The listing builds one solid part. Answer for the finished solid, in the listing's coordinates (mm). A direction names the side the tool comes from. Coordinates: 2 decimals unless noted, no trailing zeros. Order: outer loops, then holes, each group sorted by start corner. A loop starts at its lowest first (then second) coordinate and runs counter-clockwise, first axis right, second up. Notation, with made-up numbers: (-38.75, -37) -> (2.25, -37) arc R35 ccw to (2.25, -5) -> close; hole circle Ø3 at (38.5, 27.25). An arc over 180 degrees is marked (long way). One line per question, with ' | ' between items.
Autodesk Inventor part; units mm, degrees
ref_plane "YZ Plane" through (0, 0, 0) normal (1, 0, 0) x (0, 1, 0)
ref_plane "XZ Plane" through (0, 0, 0) normal (0, 1, 0) x (-1, 0, 0)
ref_plane "XY Plane" through (0, 0, 0) normal (0, 0, 1) x (1, 0, 0)
sketch "Sketch1" plane through (0, 0, 0) normal (0, 1, 0) x (-1, 0, 0)
  line L0 (0, 0) -> (125, 0)
  line L1 (125, 0) -> (125, -250)
  line L2 (125, -250) -> (0, -250)
  line L3 (0, -250) -> (0, 0)
  line L4 (62.5, -250) -> (62.5, -240)
  line L5 (62.5, -240) -> (62.5, -187.5)
  line L6 (62.5, 0) -> (62.5, -10)
  line L7 (62.5, -10) -> (62.5, -62.5018)
  dimension "d0" = 125
  dimension "d1" = 250
  dimension "d2" = 10
  dimension "d3" = 52.5
  dimension "d4" = 10
  dimension "d5" = 52.5018
extrude "Extrusion1" add sketch "Sketch1" along normal blind 100
hole "Hole1" at (-62.5, 0, -62.5018) at (-62.5, 0, -187.5) direction (0, 1, 0) diameter 105 depth 90
sketch "Sketch2" plane through (0, 0, 0) normal (0, -1, 0) x (1, 0, 0)
  line L0 (-125, -250) -> (-125, 0)
  line L1 (-125, -125) -> (-112.3, -125)
  line L2 (-112.3, -125) -> (-112.3, -121.825)
  line L3 (-112.3, -121.825) -> (-99.6, -121.825)
  line L4 (-99.6, -121.825) -> (-99.6, -128.175)
  line L5 (-99.6, -128.175) -> (-112.3, -128.175)
  line L6 (-112.3, -128.175) -> (-112.3, -121.825)
  line L7 (-112.3, -128.175) -> (-115.475, -128.175)
  line L8 (-115.475, -128.175) -> (-115.475, -121.825)
  line L9 (-115.475, -121.825) -> (-112.3, -121.825)
  line L10 (-112.3, -121.825) -> (-112.3, -128.175)
  point P0 (0, 0)
  dimension "d16" = 12.7
  dimension "d17" = 3.175
  dimension "d18" = 12.7
  dimension "d19" = 6.35
  dimension "d20" = 3.175
extrude "Extrusion2" add sketch "Sketch2" along normal blind 6.35 contours L8 L9 L2 L1 | L1 L6 L7 L8
sketch "Sketch3" plane through (0, -6.35, 0) normal (0, -1, 0) x (1, 0, 0)
  line L0 (-112.3, -128.175) -> (-112.3, -121.825)
  line L1 (-112.3, -121.825) -> (-99.6, -121.825)
  line L2 (-99.6, -121.825) -> (-99.6, -128.175)
  line L3 (-99.6, -128.175) -> (-112.3, -128.175)
  line L4 (-112.3, -128.175) -> (-112.3, -121.825)
  line L5 (-115.475, -128.175) -> (-115.475, -121.825)
  line L6 (-115.475, -121.825) -> (-112.3, -121.825)
  line L7 (-112.3, -121.825) -> (-112.3, -128.175)
  line L8 (-112.3, -128.175) -> (-115.475, -128.175)
  line L9 (-115.475, -128.175) -> (-115.475, -121.825)
  point P0 (0, 0)
  dimension "d23" = 12.7
extrude "Extrusion3" add sketch "Sketch3" along normal blind 3.175
fillet "Fillet2" radius 3.175 4 edges at (-115.475, 0, -125) (-113.8875, 0, -128.175) (-113.8875, 0, -121.825) (-112.3, 0, -125)
ref_plane "Work Plane1" through (-62.5, 0, -250) normal (-1, 0, 0) x (0, 0, 1)
mirror "Mirror1" about plane through (-62.5, 0, -250) normal (-1, 0, 0) of "Extrusion2", "Extrusion3", "Fillet2"
chamfer "Chamfer1" distance 38.1 angle 45 4 edges at (-125, 50, 0) (0, 50, 0) (0, 50, -250) (-125, 50, -250)
fillet "Fillet1" radius 6.35 16 edges at (-125, 0, -125) (-62.5, 0, 0) (0, 0, -125) (-62.5, 0, -250) (-105.95, 0, -19.05) (-19.05, 0, -19.05) (-19.05, 0, -230.95) (-105.95, 0, -230.95) (-125, 50, -38.1) (-86.9, 50, 0) (-38.1, 50, 0) (0, 50, -38.1) (0, 50, -211.9) (-86.9, 50, -250) (-125, 50, -211.9) (-38.1, 50, -250)
properties part number "Bottle Holder"
Item 1: For faces 1 (the face through (-109, -8, -128.175)), 2 (the face through (-106.2, 53.8, -230.7)), 3 (the face through (-115.475, -6, -125)), 4 (the face through (-63, 90, -187)), 5 (the face through (-62, 100, -123)), determine the directions among +Z, -Z, +X, -X, +Y, -Y from which every point of the face is accessible in a straight line to the end or side of a thin tool.
Computed values:
face 1: -Z, +X, -X, -Y | face 2: -Z, -X, +Y, -Y | face 3: +Z, -Z, -X, -Y | face 4: -Y | face 5: +Z, -Z, +X, -X, +Y
Item 2: Section C-C, the plane z = -187.5 is taken. Give the vertices of the cut face in (x, y), plus the area to 3 significant figures.
Computed values:
outline: (-125, 6.35) arc R6.35 ccw to (-118.65, 0) -> (-115, 0) -> (-115, 90) -> (-10, 90) -> (-10, 0) -> (-6.35, 0) arc R6.35 ccw to (0, 6.35) -> (0, 100) -> (-125, 100) -> close | area: 3,030 mm^2
Item 3: Section D-D, the plane x = -76 is taken. Give the vertices of the cut face in (y, z), plus the area to 3 significant figures.
Computed values:
outline: (0, -243.65) arc R6.35 ccw to (6.35, -250) -> (100, -250) -> (100, 0) -> (6.35, 0) arc R6.35 ccw to (0, -6.35) -> (0, -11.77) -> (90, -11.77) -> (90, -113.24) -> (0, -113.24) -> (0, -136.77) -> (90, -136.77) -> (90, -238.23) -> (0, -238.23) -> close | area: 6,720 mm^2
Item 4: Find the intervals of material crossed by L1, parallel to Z at x = -62.5, y = 56; L2, parallel to X at y = 43, z = -187.5; L3, parallel to Z at x = -43.5, y = 15.5, in increasing order.
Computed values:
L1: z = -250 to -240, -135 to -115, -10 to 0 | L2: x = -125 to -115, -10 to 0 | L3: z = -250 to -236.44, -138.56 to -111.44, -13.56 to 0
Item 5: Section B-B, the plane x = -62.5 is taken. Give the vertices of the cut face in (y, z).
Computed values:
outline: (0, -243.65) arc R6.35 ccw to (6.35, -250) -> (100, -250) -> (100, 0) -> (6.35, 0) arc R6.35 ccw to (0, -6.35) -> (0, -10) -> (90, -10) -> (90, -115) -> (0, -115) -> (0, -135) -> (90, -135) -> (90, -240) -> (0, -240) -> close
Item 6: Section A-A, the plane y = 13 is taken. Give the vertices of the cut face in (x, z), plus the area to 3 significant figures.
Computed values:
outline: (-125, -209.27) arc R6.35 ccw to (-123.14, -213.76) -> (-88.76, -248.14) arc R6.35 ccw to (-84.27, -250) -> (-40.73, -250) arc R6.35 ccw to (-36.24, -248.14) -> (-1.86, -213.76) arc R6.35 ccw to (0, -209.27) -> (0, -40.73) arc R6.35 ccw to (-1.86, -36.24) -> (-36.24, -1.86) arc R6.35 ccw to (-40.73, 0) -> (-84.27, 0) arc R6.35 ccw to (-88.76, -1.86) -> (-123.14, -36.24) arc R6.35 ccw to (-125, -40.73) -> close; hole circle Ø105 at (-62.5, -187.5); hole circle Ø105 at (-62.5, -62.5) | area: 11,000 mm^2
Item 7: Determine the mould class of faces 6 (the face through (-18, -9.525, -125)), 7 (the face through (-30.55, 45.63, -145.84)), 8 (the face through (-19.3, 53.8, -231.2)), 9 (the face through (-11.25, 45.63, -51.12)) for opening direction Z: pulls with the +Z half, pulls with the -Z half, needs draft (parallel to the pull), parting line crosses it, or undercut.
Computed values:
face 6: needs draft | face 7: undercut | face 8: pulls with the -Z half | face 9: undercut
Item 8: Each of these flat-tipped pins is pushed along its axis until it touches: pin 1 Ø1.6 at (y, z) = (-7.5, -124.5) entering from -X (3 decimals); pin 2 Ø7 at (x, y) = (-104, -8) entering from +Z (3 decimals); pin 3 Ø4 at (x, y) = (-107.5, 20.5) entering from +Z. Where does it stop, or does it pass through?
Computed values:
pin 1: stops at x = -115.475 | pin 2: stops at z = -121.825 | pin 3: stops at z = -18.6
